The model under review builds one solid part; all positions refer to its coordinate system, in mm. A direction names the side the tool comes from. Round coordinates to 2 decimals unless told otherwise and drop trailing zeros. Write each loop counter-clockwise with the first axis right and the second up, starting at its lowest first coordinate (ties: lowest second). Pieces come first, ordered by that corner, then holes.
Item 1: Clearance check with flat-ended pins moving along their axes: pin 1 Ø0.6 at (x, y) = (41, 32.5) entering from +Z; pin 2 Ø1 at (y, z) = (23.5, -17.5) entering from -X. State where each tip first meets the part, or that it passes through.
Item 2: Machinability: for faces 1 (the face through (20, 30, -22)), 2 (the face through (-1, 30, -18.5)), 3 (the face through (40, 30, -17)), which of the approach directions +Z, -Z, +X, -X, +Y, -Y give a long, thin tool a straight path to every point of the face, cutting with its end or side? Answer none if there is none.
Item 3: Add section A-A (y = 36). Give the boundary of the cut face in (x, z).
Item 4: Add section B-B (z = -17). Give the boundary of the cut face in (x, y), plus the area to 3 significant figures.
Item 5: To check wall thickness, follow L1, parallel to X at y = 14, z = -16.5. State the ranges of the line that lie inside material, in increasing order.
```python
from build123d import *

# Parameters (mm, degrees)
BOX003_W     = 44
BOX003_H     = 40
BOX003_DEPTH = 3.5
BOX002_W     = 40
BOX002_H     = 40
BOX002_DEPTH = 3.3


with BuildPart() as radiator:
    # Box003 → Box003 (new body)
    with BuildSketch(Plane(origin=(-2, 0, -3.5), x_dir=(1, 0, 0), z_dir=(0, 0, 1))):
        with Locations((22, 20)):
            Rectangle(BOX003_W, BOX003_H)
    extrude(amount=BOX003_DEPTH)


with BuildPart() as obj1:
    # Box002 → Box002 (new body)
    with BuildSketch(Plane.XY):
        with Locations((20, 20)):
            Rectangle(BOX002_W, BOX002_H)
    extrude(amount=BOX002_DEPTH)

    # Fusion003: union radiator
    add(radiator.part)


with BuildPart() as obj1_1:
    # Fusion003 placement: moved
    add(obj1.part.moved(Location((0, 10, -18.5))))


solid = obj1_1.part
```
Numbers:
1. pin 1: stops at z = -18.5
1. pin 2: stops at x = 0
2. face 1: -Z, +X, -X, +Y, -Y
2. face 2: +Z, -X, +Y, -Y
2. face 3: +Z, +X, +Y, -Y
3. outline: (-2, -22) - (42, -22) - (42, -18.5) - (40, -18.5) - (40, -15.2) - (0, -15.2) - (0, -18.5) - (-2, -18.5) - close
4. outline: (0, 10) - (40, 10) - (40, 50) - (0, 50) - close
4. area: 1,600 mm2
5. L1: x = 0 to 40
